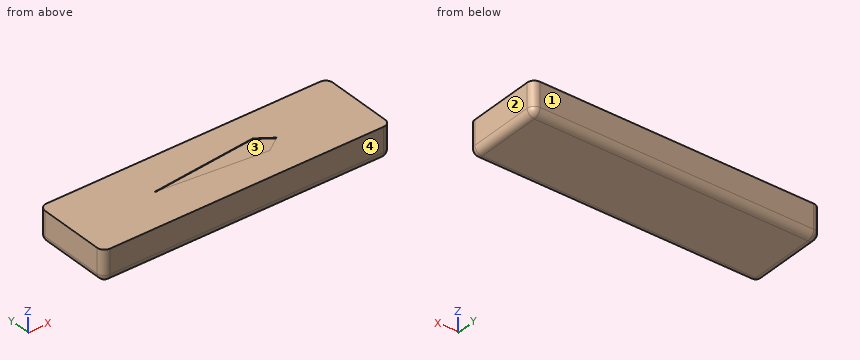
from build123d import *

# Parameters (mm, degrees)
F0_W     = 201
F0_H     = 56
F1_DEPTH = 22
F2_R     = 5
F3_DEPTH = 21.6


with BuildPart() as f1:
    # F0 (on Top) → F1 (new body)
    with BuildSketch(Plane.XY):
        with Locations((34.910782, -1.85752)):
            Rectangle(F0_W, F0_H)
        Polygon((67.267462, -9.29118), (-7.982538, -1.79118), (67.267462, 5.70882), (78.017462, -1.79118), align=None, mode=Mode.SUBTRACT)
    extrude(amount=F1_DEPTH)

    # F2
    f2_edges = [f1.edges().sort_by_distance(p)[0] for p in [
        (34.910782, 26.14248, 0),
        (-65.589218, -1.85752, 0),
        (34.910782, -29.85752, 0),
        (135.410782, -1.85752, 0),
        (135.410782, 26.14248, 11),
        (-65.589218, 26.14248, 11),
        (-65.589218, -29.85752, 11),
        (135.410782, -29.85752, 11),
    ]]
    fillet(f2_edges, radius=F2_R)

    # F0 (on Top) → F3 (join)
    with BuildSketch(Plane.XY):
        Polygon((67.267462, 5.70882), (-7.982538, -1.79118), (67.267462, -9.29118), (78.017462, -1.79118), align=None)
    extrude(amount=F3_DEPTH)


solid = f1.part
Can you work these out from the model? Positions are in its coordinate system, mm. Face numbers are marked on the shaded views. Coordinates: 2 decimals unless noted, no trailing zeros. Loops run counter-clockwise (first coordinate to the right, second up) from the corner with the lowest first, then second, coordinate; pieces in that order, holes last. Notation, with made-up numbers: M 69.5,10.25 L 84.5,10.25 A18 cw 84.5,25.25 Z; hole C -20.75,8.5 d4. An arc over 180 degrees is marked long. Return JSON: item names as keys, results as strings. Group by question number.
Item 1: If I drill on L1, parallel to Z at x = -37.5, y = -25.5; L2, parallel to Z at x = 46, y = 0; L3, parallel to X at y = -6, z = 2.5, over which ranges is the centre line in solid material (lowest first)? Write a range as from..to.
Item 2: I'm going to push a flat-ended pin straight in: pin 1 Ø7.5 at (x, y) = (40, -1) entering from +Z. Where does the tip first touch, or does it pass through?
Item 3: Thinking about a two-plate mould opening in Y: for the marked faces 1, 2, 3 and 4, which applies, released by +Y, released by -Y, zero draft, split by the parting line, or undercut?
Item 4: Imagine slicing it at A-A (z = 3.25). Please give me the cut outline in (x, y), and give its area (3 significant figures).
Verdict:
{
 "1": {"L1": "z = 0.04..22", "L2": "z = 0..21.6", "L3": "x = -64.92..134.74"},
 "2": {"pin 1": "stops at z = 21.6"},
 "3": {"face 1": "released by +Y", "face 2": "zero draft", "face 3": "undercut", "face 4": "released by -Y"},
 "4": {"outline": "M -65.27,-24.86 A4.68 ccw -60.59,-29.54 L 130.41,-29.54 A4.68 ccw 135.09,-24.86 L 135.09,21.14 A4.68 ccw 130.41,25.83 L -60.59,25.83 A4.68 ccw -65.27,21.14 Z", "area": "11,100 mm^2"}
}
